Geometry: final body of the model. Coordinates: model frame, mm. Coordinates: 2 decimals unless noted, no trailing zeros. Order: outer loops, then holes, each group sorted by start corner. A loop starts at its lowest first (then second) coordinate and runs counter-clockwise, first axis right, second up. Notation, with made-up numbers: (-21, 75) -> (16, 75) arc R24 ccw to (16, 85) -> close; hole circle Ø1 at (2.25, 77.5). An arc over 180 degrees is marked (long way). Answer in a Markdown table with one row per item. Add a question column.
1) Section query D-D on y = 6. Return the cut outline in (x, z), then the cut area to 3 significant figures.
2) Ray query, line 1 (X direction, y = 2.25, z = 0.3); line 2 (Y direction, x = -3, z = 0.9); line 3 (Y direction, x = -6.5, z = 0.7). Return the intervals inside material, ascending. Write a range as from..to.
3) Contact query for flat-ended pins moving along their axis: P1, Ø0.5, axis at x = -7.5, z = 0.5, coming from the +Y side; P2, Ø0.5, axis at x = -6.5, z = 0.5, coming from the -Y side; P3, Ø0.5, axis at x = 2.5, z = 0.5, coming from the +Y side. Output: stop coordinate, or through.
4) Section query B-B on z = 0.3. Count the separate pieces of the cut face and the enclosed holes in it, then the cut area to 3 significant figures.
5) Section query A-A on x = 0. Return the cut outline in (y, z).
6) Pull-direction query (Y, two-part tool) for faces 1 (the face through (-2, 0, 1)), 2 (the face through (-7.5, 0.5, 0.5)); classes: +Y half, -Y half, draft (parallel to the pull), parting line (faces both ways), or undercut.
```python
from build123d import *

# Parameters (mm, degrees)
F0_W     = 9.5
F0_H     = 1
F0_W_2   = 1
F0_H_2   = 9.5
F1_DEPTH = 1
F2_R     = 10.25
F2_R_2   = 9.75
F2_R_3   = 5.25
F2_R_4   = 4.75
F3_DEPTH = 1
F4_R     = 1
F5_DEPTH = 25


with BuildPart() as f1:
    # F0 (on Top) → F1 (new body)
    with BuildSketch(Plane.XY):
        with Locations((-5.25, 0)):
            Rectangle(F0_W, F0_H)
        with Locations((0, 5.25)):
            Rectangle(F0_W_2, F0_H_2)
        with Locations((5.25, 0)):
            Rectangle(F0_W, F0_H)
        with Locations((0, -5.25)):
            Rectangle(F0_W_2, F0_H_2)
    extrude(amount=F1_DEPTH)

    # F2 (on Top) → F3 (join)
    with BuildSketch(Plane.XY):
        Circle(F2_R)
        Circle(F2_R_2, mode=Mode.SUBTRACT)
        Circle(F2_R_3)
        Circle(F2_R_4, mode=Mode.SUBTRACT)
    extrude(amount=F3_DEPTH)

    # F4 (on Top) → F5 (cut)
    with BuildSketch(Plane.XY):
        Circle(F4_R)
    extrude(amount=F5_DEPTH, mode=Mode.SUBTRACT)


solid = f1.part
```
Result:
| question | item | result |
|---|---|---|
| 1 | outline | (-8.31, 0) -> (-7.69, 0) -> (-7.69, 1) -> (-8.31, 1) -> close; (-0.5, 0) -> (0.5, 0) -> (0.5, 1) -> (-0.5, 1) -> close; (7.69, 0) -> (8.31, 0) -> (8.31, 1) -> (7.69, 1) -> close |
| 1 | area | 2.25 mm2 |
| 2 | line 1 | -10..-9.49, -4.74..-4.18, -0.5..0.5, 4.18..4.74, 9.49..10 |
| 2 | line 2 | -9.8..-9.28, -4.31..-3.68, -0.5..0.5, 3.68..4.31, 9.28..9.8 |
| 2 | line 3 | -7.93..-7.27, -0.5..0.5, 7.27..7.93 |
| 3 | P1 | y = 7.25 |
| 3 | P2 | y = -8.12 |
| 3 | P3 | y = 10 |
| 4 | separate pieces | 1 |
| 4 | enclosed holes | 5 |
| 4 | area | 80.3 mm2 |
| 5 | outline | (-10.25, 0) -> (-1, 0) -> (-1, 1) -> (-10.25, 1) -> close; (1, 0) -> (10.25, 0) -> (10.25, 1) -> (1, 1) -> close |
| 6 | face 1 | draft |
| 6 | face 2 | undercut |
